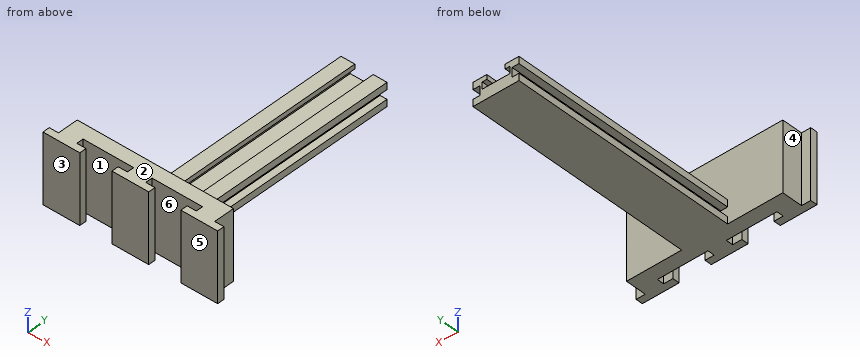
Autodesk Inventor part; units mm, degrees
ref_plane "YZ Plane" through (0, 0, 0) normal (1, 0, 0) x (0, 1, 0)
ref_plane "XZ Plane" through (0, 0, 0) normal (0, 1, 0) x (-1, 0, 0)
ref_plane "XY Plane" through (0, 0, 0) normal (0, 0, 1) x (1, 0, 0)
sketch "Sketch1" plane through (0, 0, 0) normal (0, 0, 1) x (1, 0, 0)
  line L0 (-300, 0) -> (300, 0)
  line L1 (300, 0) -> (300, 50)
  line L2 (-300, 50) -> (-300, 0)
  line L3 (-20, 50) -> (-20, 35)
  line L4 (-20, 35) -> (-40, 35)
  line L5 (-40, 35) -> (-40, 20)
  line L6 (-40, 20) -> (40, 20)
  line L7 (40, 20) -> (40, 35)
  line L8 (40, 35) -> (20, 35)
  line L9 (20, 35) -> (20, 50)
  line L10 (-75, 159.793) -> (-75, -97.8722) construction
  line L11 (75, 159.793) -> (75, -92.8199) construction
  line L12 (-110, 20) -> (-190, 20)
  line L13 (-190, 20) -> (-190, 35)
  line L14 (-110, 35) -> (-110, 20)
  line L15 (-130, 35) -> (-110, 35)
  line L16 (-130, 50) -> (-130, 35)
  line L17 (-170, 35) -> (-170, 50)
  line L18 (-190, 35) -> (-170, 35)
  line L19 (170, 50) -> (170, 35)
  line L20 (170, 35) -> (190, 35)
  line L21 (190, 35) -> (190, 20)
  line L22 (190, 20) -> (110, 20)
  line L23 (110, 20) -> (110, 35)
  line L24 (110, 35) -> (130, 35)
  line L25 (130, 35) -> (130, 50)
  line L26 (-20, 50) -> (-130, 50)
  line L27 (-170, 50) -> (-300, 50)
  line L28 (300, 50) -> (170, 50)
  line L29 (130, 50) -> (20, 50)
  line L30 (170, 35) -> (170, 80)
  line L31 (170, 80) -> (-170, 80)
  line L32 (-170, 80) -> (-170, 35)
  point P0 (0, 0)
  point P1 (0, 0)
  dimension "d0" = 300
  dimension "d1" = 600
  dimension "d2" = 50
  dimension "d3" = 50
  dimension "d4" = 20
  dimension "d5" = 20
  dimension "d6" = 20
  dimension "d7" = 20
  dimension "d8" = 30
  dimension "d9" = 15
  dimension "d10" = 15
  dimension "d11" = 75
  dimension "d12" = 75
  dimension "d13" = 15
  dimension "d14" = 109.793
  dimension "d15" = 142.8199
  dimension "d16" = 109.793
  dimension "d17" = 147.8722
  dimension "d18" = 45
sketch "Sketch2" plane through (0, 0, 0) normal (0, 0, 1) x (1, 0, 0)
  point P0 (0, 0)
extrude "Extrusion1" add sketch "Sketch1" along normal blind 150 contours L32 L31 L30 L19 L20 L21 L22 L23 L24 L25 L29 L9 L8 L7 L6 L5 L4 L3 L26 L16 L15 L14 L12 L13 L18 L17
sketch "Sketch3" plane through (-170, 80, 0) normal (0, 1, 0) x (1, 0, 0)
  line L0 (170, 0) -> (130, 0)
  line L1 (130, 0) -> (130, -50) construction
  line L2 (130, -50) -> (170, -50)
  line L3 (340, 0) -> (0, 0)
  line L4 (170, -50) -> (210, -50)
  line L5 (210, -50) -> (210, 0) construction
  line L6 (210, 0) -> (170, 0)
  line L7 (120, -50) -> (220, -50)
  line L8 (220, -50) -> (220, 0)
  line L9 (220, 0) -> (120, 0)
  line L10 (120, 0) -> (120, -50)
  line L11 (120, -50) -> (220, 0) construction
  line L12 (220, -50) -> (120, 0) construction
  point P0 (170, -25)
  dimension "d21" = 40
  dimension "d22" = 50
  dimension "d23" = 40
  dimension "d36" = 100
extrude "Extrusion2" add sketch "Sketch3" along normal blind 500
sketch "Sketch5" plane through (-170, 580, 0) normal (0, 1, 0) x (1, 0, 0)
  line L0 (150, 0) -> (150, -150)
  line L1 (190, -60) -> (150, -60)
  line L2 (150, -60) -> (150, -40)
  line L3 (150, -40) -> (190, -40) construction
  line L4 (190, -40) -> (190, -60)
  line L5 (220, -50) -> (120, -50)
  line L6 (190, -60) -> (150, -40) construction
  line L7 (150, -60) -> (190, -40) construction
  line L8 (150, -40) -> (140, -40)
  line L9 (140, -40) -> (140, -25)
  line L10 (140, -25) -> (200, -25)
  line L11 (200, -25) -> (200, -40)
  line L12 (200, -40) -> (190, -40)
  point P0 (170, 0)
  point P1 (170, -50)
  point P2 (210, -50)
  point P3 (130, -50)
  point P4 (170, -50)
  dimension "d26" = 10
  dimension "d27" = 15
  dimension "d28" = 60
  dimension "d31" = 20
extrude "Extrusion3" cut sketch "Sketch5" against normal blind 500
sketch "Sketch6" plane through (-170, 580, 0) normal (0, 1, 0) x (1, 0, 0)
  line L0 (130, 0) -> (130, -150)
  line L1 (150, 0) -> (150, -150)
  line L2 (135, -30) -> (135, -20)
  line L3 (170, 0) -> (170, -54.7641) construction
  line L4 (120, -50) -> (120, 0)
  line L5 (120, -20) -> (120, -30)
  line L6 (220, 0) -> (220, -50)
  line L7 (135, -20) -> (135, -15)
  line L8 (135, -15) -> (120, -15)
  line L9 (120, -30) -> (120, -35)
  line L10 (120, -35) -> (135, -35)
  line L11 (135, -35) -> (135, -30)
  line L12 (120, -15) -> (120, -20)
  line L13 (205, -30) -> (205, -20)
  line L14 (220, -50) -> (220, 0)
  line L15 (205, -20) -> (205, -15)
  line L16 (205, -15) -> (220, -15)
  line L17 (220, -30) -> (220, -35)
  line L18 (220, -35) -> (205, -35)
  line L19 (205, -35) -> (205, -30)
  point P0 (130, -35)
  point P1 (130, -15)
  dimension "d38" = 5
  dimension "d39" = 15
extrude "Extrusion4" cut sketch "Sketch6" against normal blind 500
properties part number "Clamp jaw handle"
Work out the finished part from the listing and answer in its coordinate system (mm). Face numbers are marked on the shaded views. A direction names the side the tool comes from. Round coordinates to 2 decimals unless told otherwise and drop trailing zeros. Write each loop counter-clockwise with the first axis right and the second up, starting at its lowest first coordinate (ties: lowest second). Pieces come first, ordered by that corner, then holes. Notation, with made-up numbers: (2, 34.25) -> (27, 34.25) arc R9 cw to (27, 42.25) -> close; hole circle Ø4 at (39.25, 2). An arc over 180 degrees is marked (long way). Write each question's results on one line, items separated by ' | '.
Q1. Section A-A, the plane x = -121.5 is taken. Write down the section's boundary in (y, z), then the cut area to 3 significant figures.
Data:
outline: (20, 0) -> (35, 0) -> (35, 150) -> (20, 150) -> close; (50, 0) -> (80, 0) -> (80, 150) -> (50, 150) -> close | area: 6,750 mm^2
Q2. Straight lines are drawn through the part: line 1 along Y through (x, z) = (-31.5, 117); line 2 along X through (y, z) = (400.5, 42.5); line 3 along Z through (x, y) = (-40, 396.5). For each, find the intervals that lie inside material, in ascending order. Write a range as [from, to].
Data:
line 1: [20, 35], [50, 80] | line 2: [-50, -20], [20, 50] | line 3: [0, 15], [35, 50]
Q3. Section D-D, the plane x = 138 is taken. Write down the section's boundary in (y, z).
Data:
outline: (20, 0) -> (80, 0) -> (80, 150) -> (20, 150) -> close
Q4. Which of the six approach directions +Z, -Z, +X, -X, +Y, -Y give full straight-line access (tool end or side, diameter ignored) to the marked faces 4, 5 and 6?
Data:
face 4: +Z, -Z, -X, +Y | face 5: +Z, -Z, +X, -X, -Y | face 6: +Z, -Z
Q5. Flat-ended cylindrical pins translate along their axes: P1, Ø22.5, axis at y = 64, z = 68.5, coming from the -X side; P2, Ø8, axis at y = 302, z = 44, coming from the -X side; P3, Ø6, axis at x = 177, z = 106.5, coming from the +Y side; P4, Ø6, axis at x = -46, y = 315.5, coming from the -Z side. Find the tip coordinate at first contact, or state that the pin passes through.
Data:
P1: x = -170 | P2: x = -50 | P3: y = 35 | P4: z = 0
Q6. Section C-C, the plane z = 63.5 is taken. Write down the section's boundary in (x, y), then the cut area to 3 significant figures.
Data:
outline: (-190, 20) -> (-110, 20) -> (-110, 35) -> (-130, 35) -> (-130, 50) -> (-20, 50) -> (-20, 35) -> (-40, 35) -> (-40, 20) -> (40, 20) -> (40, 35) -> (20, 35) -> (20, 50) -> (130, 50) -> (130, 35) -> (110, 35) -> (110, 20) -> (190, 20) -> (190, 35) -> (170, 35) -> (170, 80) -> (-170, 80) -> (-170, 35) -> (-190, 35) -> close | area: 15,600 mm^2
Q7. Determine the mould class of the marked faces 1, 2 and 3 for opening direction Y: released by +Y, released by -Y, zero draft, split by the parting line, or undercut.
Data:
face 1: undercut | face 2: zero draft | face 3: released by -Y
Q8. Section B-B, the plane y = 340 is taken. Write down the section's boundary in (x, z), then the cut area to 3 significant figures.
Data:
outline: (-50, 0) -> (50, 0) -> (50, 15) -> (35, 15) -> (35, 35) -> (50, 35) -> (50, 50) -> (20, 50) -> (20, 40) -> (30, 40) -> (30, 25) -> (-30, 25) -> (-30, 40) -> (-20, 40) -> (-20, 50) -> (-50, 50) -> (-50, 35) -> (-35, 35) -> (-35, 15) -> (-50, 15) -> close | area: 3,100 mm^2
